For this review, use the dimensioned drawing (mm, ordinates from the lowest corner) and the shaded views. A direction names the side the tool comes from. Coordinates: 2 decimals unless noted, no trailing zeros. Write each loop counter-clockwise with the first axis right and the second up, starting at its lowest first coordinate (ties: lowest second). Pieces come first, ordered by that corner, then holes. Notation, with made-up numbers: (62, 53) - (77, 53) arc R19 ccw to (77, 81) - close; hole circle Ø1 at (74.5, 52). An arc over 180 degrees is marked (long way). Answer as a JSON object with one key per item and string values.
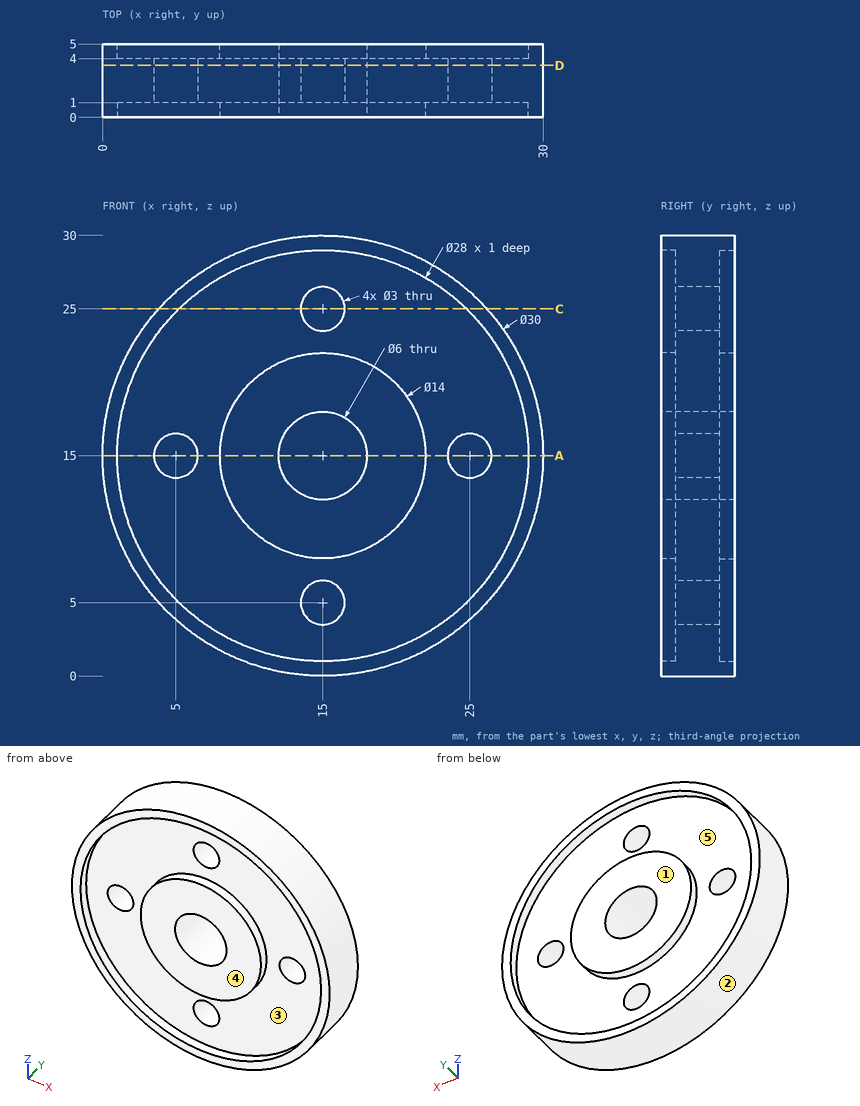
(1) Take a section at A-A, the plane z = 15. Give the number of separate pieces and of enclosed holes in the cut face, and give its area (3 significant figures).
Solved:
{"separate pieces": "4", "enclosed holes": "0", "area": "74.0 mm^2"}
(2) For pin 1 (3 mm diameter, centred on y = 3, z = 4.5, fed in from -X); pin 2 (1.5 mm diameter, centred on x = 3, z = 8, fed in from +Y); pin 3 (5 mm diameter, centred on x = 15, z = 25, fed in from +Y); pin 4 (5 mm diameter, centred on x = 25, z = 15, fed in from -Y), all flat-tipped, find the tip position at first contact; note any pin that passes through.
Solved:
{"pin 1": "stops at x = 3", "pin 2": "stops at y = 5", "pin 3": "stops at y = 4", "pin 4": "stops at y = 1"}
(3) The part is to be moulded in two halves that separate along X. For the marked faces 1, 2 and 3, say which applies: pulls with the +X half, pulls with the -X half, needs draft (parallel to the pull), parting line crosses it, or undercut.
Solved:
{"face 1": "needs draft", "face 2": "parting line crosses it", "face 3": "undercut"}
(4) Take a section at C-C, the plane z = 25. Write out the cut boundary in (x, y).
Solved:
{"outline": "(3.82, 0) - (5.2, 0) - (5.2, 1) - (13.5, 1) - (13.5, 4) - (5.2, 4) - (5.2, 5) - (3.82, 5) - close; (16.5, 1) - (24.8, 1) - (24.8, 0) - (26.18, 0) - (26.18, 5) - (24.8, 5) - (24.8, 4) - (16.5, 4) - close"}
(5) To check wall thickness, follow line 1 (Z direction, x = 15, y = 2.5); line 2 (X direction, y = 4.7, z = 15). State the ranges of each line that lie inside material, in increasing order. Write a range as from..to.
Solved:
{"line 1": "z = 0..3.5, 6.5..12, 18..23.5, 26.5..30", "line 2": "x = 0..1, 8..12, 18..22, 29..30"}
(6) Tool access review of the marked faces 4 and 5: name each direction out of +Z, -Z, +X, -X, +Y, -Y from which nothing blocks a thin tool from reaching the whole face with its end or side.
Solved:
{"face 4": "+Z, -Z, +X, -X, -Y", "face 5": "+Y"}
(7) Take a section at D-D, the plane y = 3.55. Write out the cut boundary in (x, z), and give its area (3 significant figures).
Solved:
{"outline": "circle Ø30 at (15, 15); hole circle Ø3 at (5, 15); hole circle Ø6 at (15, 15); hole circle Ø3 at (15, 5); hole circle Ø3 at (15, 25); hole circle Ø3 at (25, 15)", "area": "650 mm^2"}
